For this review, use the dimensioned drawing (mm, ordinates from the lowest corner) and the shaded views. A direction names the side the tool comes from. Give positions to 0.01 mm unless a question says otherwise; leave off trailing zeros. Order: outer loops, then holes, each group sorted by start corner. A loop starts at its lowest first (then second) coordinate and runs counter-clockwise, first axis right, second up. Notation, with made-up numbers: M 24,-39.5 L 57,-39.5 A14 cw 57,-26.5 Z; hole C 12.5,28.25 d5. An arc over 180 degrees is marked long. Answer as CSV lines item,"result". Start each with the question number.
1. We need section A-A, the plane z = 23. Give the boundary of the cut face in (x, y), and give its area (3 significant figures).
2. We need section C-C, the plane y = 6.75. Give the boundary of the cut face in (x, z).
3. For line 1 along Y through (x, z) = (27, 25); line 2 along X through (y, z) = (9.25, 19.5); line 3 along X through (y, z) = (3.25, 10), list the stretches that pass through material, from the lowest coordinate up.
4. Mouldability with a two-part tool opening along Y and no side actions: class the marked faces 1, 2 and 3 as pulls with the +Y half, pulls with the -Y half, needs draft (parallel to the pull), parting line crosses it, or undercut.
5. Machinability: for the marked faces 4 and 5, which of the approach directions +Z, -Z, +X, -X, +Y, -Y give a long, thin tool a straight path to every point of the face, cutting with its end or side? Answer none if there is none.
6. We need section B-B, the plane x = 10. Give the boundary of the cut face in (y, z).
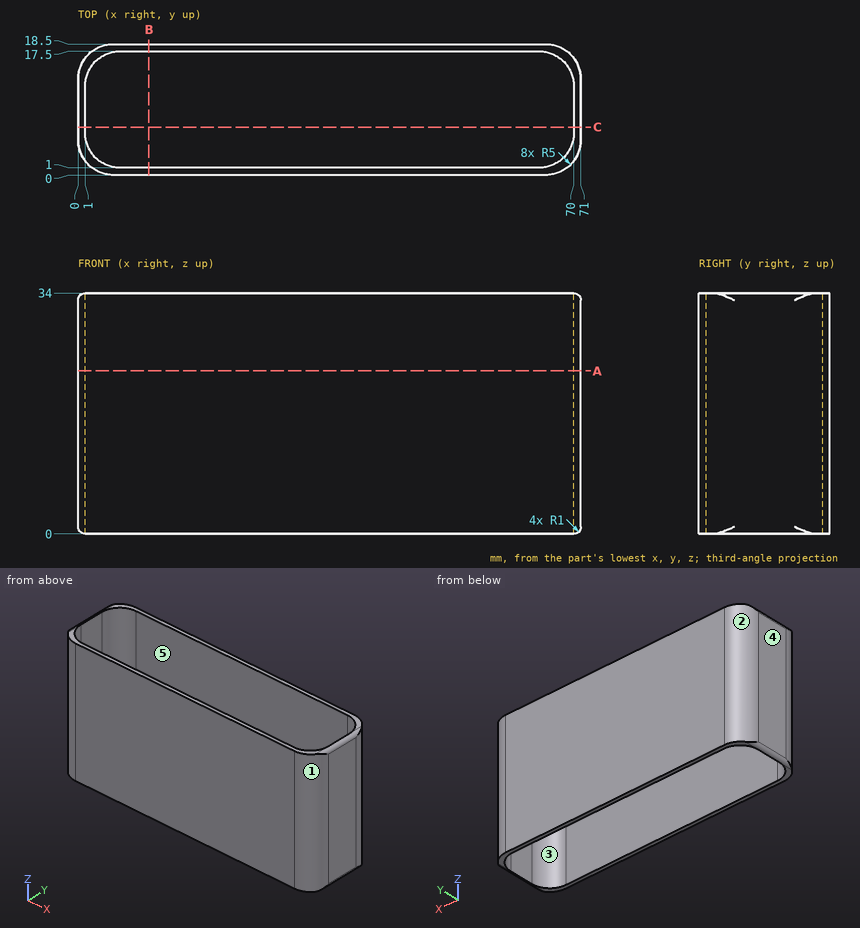
Result set:
1,outline,"M 0,5 A5 ccw 5,0 L 66,0 A5 ccw 71,5 L 71,13.5 A5 ccw 66,18.5 L 5,18.5 A5 ccw 0,13.5 Z; hole M 1,6 A5 ccw 6,1 L 65,1 A5 ccw 70,6 L 70,12.5 A5 ccw 65,17.5 L 6,17.5 A5 ccw 1,12.5 Z"
1,area,"175 mm2"
2,outline,"M 0,1 A1 ccw 1,0 L 1,34 A1 ccw 0,33 Z; M 70,0 A1 ccw 71,1 L 71,33 A1 ccw 70,34 Z"
3,line 1,"0 to 1, 17.5 to 18.5"
3,line 2,"0 to 1, 70 to 71"
3,line 3,"0.32 to 1.82, 69.18 to 70.68"
4,face 1,"pulls with the -Y half"
4,face 2,"pulls with the +Y half"
4,face 3,"undercut"
5,face 4,"+Z, -Z, -X, +Y, -Y"
5,face 5,"+Z, -Z"
6,outline,"M 0,0 L 1,0 L 1,34 L 0,34 Z; M 17.5,0 L 18.5,0 L 18.5,34 L 17.5,34 Z"
